Geometry: final body of the model. Coordinates: model frame, mm. Face numbers are marked on the shaded views. A direction names the side the tool comes from. Round coordinates to 2 decimals unless told otherwise and drop trailing zeros. Loops run counter-clockwise (first coordinate to the right, second up) from the corner with the lowest first, then second, coordinate; pieces in that order, holes last. Notation, with made-up numbers: (-5.5, 48.25) - (-1.5, 48.25) arc R23 ccw to (-1.5, 63.25) - close; hole circle Ø2 at (12, -3). An arc over 180 degrees is marked (long way). Answer as CSV lines item,"result".
from build123d import *

# Parameters (mm, degrees)
F0_R     = 32.5
F1_DEPTH = 2.5
F2_W     = 10
F2_H     = 14.76
F2_W_2   = 40
F3_DEPTH = 11
F4_W     = 10
F4_H     = 14.76
F5_DEPTH = 20
F6_R     = 2.25
F7_DEPTH = 25.4


with BuildPart() as f1:
    # F0 (on Top) → F1 (new body)
    with BuildSketch(Plane.XY):
        Circle(F0_R)
    extrude(amount=F1_DEPTH)

    # F2 (on face) → F3 (join)
    with BuildSketch(Plane.XY.offset(2.5)):
        with Locations((25, 0)):
            Rectangle(F2_W, F2_H)
        Rectangle(F2_W_2, F2_H)
        with Locations((-25, 0)):
            Rectangle(F2_W, F2_H)
    extrude(amount=F3_DEPTH)

    # F4 (on face) → F5 (join)
    with BuildSketch(Plane.XY.offset(13.5)):
        with Locations((25, 0)):
            Rectangle(F4_W, F4_H)
        with Locations((-25, 0)):
            Rectangle(F4_W, F4_H)
    extrude(amount=F5_DEPTH)

    # F6 (on face) → F7 (cut)
    with BuildSketch(Plane.XZ.offset(7.38)):
        with Locations((-24.5, 17.5)):
            Circle(F6_R)
        with Locations((-24.5, 29.5)):
            Circle(F6_R)
        with Locations((24.5, 17.5)):
            Circle(F6_R)
        with Locations((24.5, 29.5)):
            Circle(F6_R)
    extrude(amount=-F7_DEPTH, mode=Mode.SUBTRACT)


solid = f1.part
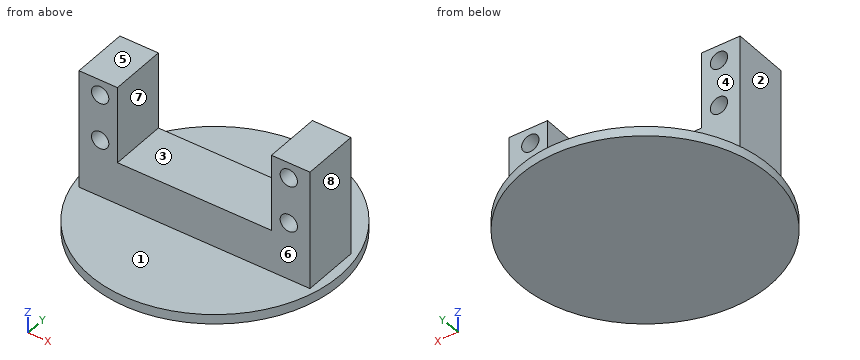
(1) Section B-B (y = 0). Output: boundary loops of the cut face in (x, z).
Findings below:
outline,"(-32.5, 0) - (32.5, 0) - (32.5, 2.5) - (30, 2.5) - (30, 33.5) - (20, 33.5) - (20, 13.5) - (-20, 13.5) - (-20, 33.5) - (-30, 33.5) - (-30, 2.5) - (-32.5, 2.5) - close; hole circle Ø4.5 at (-24.5, 17.5); hole circle Ø4.5 at (-24.5, 29.5); hole circle Ø4.5 at (24.5, 17.5); hole circle Ø4.5 at (24.5, 29.5)"
(2) Draft query along X for the marked faces 1, 2 and 3. Return one class per face: pulls with the +X half, pulls with the -X half, needs draft (parallel to the pull), parting line crosses it, or undercut.
Findings below:
face 1,"needs draft"
face 2,"pulls with the -X half"
face 3,"undercut"
(3) Section A-A (z = 24). Output: boundary loops of the cut face in (x, y), and give its area (3 significant figures).
Findings below:
outline,"(-30, -7.38) - (-20, -7.38) - (-20, 7.38) - (-30, 7.38) - close; (20, -7.38) - (30, -7.38) - (30, 7.38) - (20, 7.38) - close"
area,"295 mm2"
(4) Section C-C (x = -24.5). Output: boundary loops of the cut face in (y, z).
Findings below:
outline,"(-21.35, 0) - (21.35, 0) - (21.35, 2.5) - (7.38, 2.5) - (7.38, 15.25) - (-7.38, 15.25) - (-7.38, 2.5) - (-21.35, 2.5) - close; (-7.38, 19.75) - (7.38, 19.75) - (7.38, 27.25) - (-7.38, 27.25) - close; (-7.38, 31.75) - (7.38, 31.75) - (7.38, 33.5) - (-7.38, 33.5) - close"
(5) Material intervals for line 1 along X through (y, z) = (-4, 17); line 2 along Z through (x, y) = (-24.5, -3.25); line 3 along X through (y, z) = (-5, 24), sorted ascending.
Findings below:
line 1,"-30 to -26.69, -22.31 to -20, 20 to 22.31, 26.69 to 30"
line 2,"0 to 15.25, 19.75 to 27.25, 31.75 to 33.5"
line 3,"-30 to -20, 20 to 30"
(6) Section D-D (z = 17.5). Output: boundary loops of the cut face in (x, y).
Findings below:
outline,"(-30, -7.38) - (-26.75, -7.38) - (-26.75, 7.38) - (-30, 7.38) - close; (-22.25, -7.38) - (-20, -7.38) - (-20, 7.38) - (-22.25, 7.38) - close; (20, -7.38) - (22.25, -7.38) - (22.25, 7.38) - (20, 7.38) - close; (26.75, -7.38) - (30, -7.38) - (30, 7.38) - (26.75, 7.38) - close"
(7) Access query for the marked faces 4, 5, 6, 7 and 8. Directions: +Z, -Z, +X, -X, +Y, -Y. A direction counts if a zero-diameter tool reaches every point of the face in a straight line with its end or side. Return the directions, or none.
Findings below:
face 4,"+Z, +X, -X, +Y"
face 5,"+Z, +X, -X, +Y, -Y"
face 6,"+Z, +X, -X, -Y"
face 7,"+Z, +Y, -Y"
face 8,"+Z, +X, +Y, -Y"
(8) Pin query (flat end, axial travel): P1, Ø3.5, axis at x = -24.5, z = 17.5, coming from the +Y side; P2, Ø12, axis at x = -15, y = 1, coming from the -Z side; P3, Ø7, axis at x = -24.5, z = 29.5, coming from the -Y side; P4, Ø6, axis at x = 8.5, y = -22.5, coming from the +Z side. Return the tip coordinate at first contact, or that it passes through.
Findings below:
P1,"through"
P2,"z = 0"
P3,"y = -7.38"
P4,"z = 2.5"
